Solid Edge part; units mm, degrees
sketch "Sketch1" plane through (0, 0, 0) normal (0, 0, 1) x (1, 0, 0)
  line L0 (-60, -45) -> (60, -45)
  line L1 (60, -45) -> (60, 45)
  line L2 (60, 45) -> (-60, 45)
  line L3 (-60, 45) -> (-60, -45)
extrude "Protrusion1" add sketch "Sketch1" along normal blind 15
sketch "Sketch2" plane through (0, 0, 0) normal (0, 0, -1) x (1, 0, 0)
  circle A0 centre (0, 0) radius 26
extrude "VaciadoExtruido_1" cut sketch "Sketch2" against normal blind 4
sketch "Sketch3" plane through (0, 0, 4) normal (0, 0, -1) x (1, 0, 0)
  line L0 (-12, -12) -> (12, -12)
  line L1 (12, -12) -> (12, 12)
  line L2 (12, 12) -> (-12, 12)
  line L3 (-12, 12) -> (-12, -12)
  dimension "D1" = 12
  dimension "D2" = 12
extrude "Cutout1" cut sketch "Sketch3" against normal through all
fillet "Redondeo_1" radius 2 4 edges at (-12, 12, 9.5) (-12, -12, 9.5) (12, -12, 9.5) (12, 12, 9.5)
chamfer "Chaflán_1" distance 5 angle 45 4 edges at (-60, 45, 7.5) (-60, -45, 7.5) (60, -45, 7.5) (60, 45, 7.5)
hole "Agujero_1" at (0, 38, 15) direction (0, 0, -1) diameter 8 end up to next start chamfer 0.5 start chamfer angle 45 end chamfer 0.5 end chamfer angle 45
hole "Hole1" at (0, -38, 15) direction (0, 0, -1) diameter 8 end up to next start chamfer 0.5 start chamfer angle 45 end chamfer 0.5 end chamfer angle 45
hole "Agujero_3" at (45.4585, 38, 15) direction (0, 0, -1) diameter 4.917 end through all start chamfer 0.5 start chamfer angle 45 end chamfer 0.5 end chamfer angle 45 thread major 6 thread length 2
hole "Hole2" at (43, -38, 15) direction (0, 0, -1) diameter 4.917 end through all start chamfer 0.5 start chamfer angle 45 end chamfer 0.5 end chamfer angle 45 thread major 6 thread length 2
hole "Hole3" at (-43, -38, 15) direction (0, 0, -1) diameter 4.917 end through all start chamfer 0.5 start chamfer angle 45 end chamfer 0.5 end chamfer angle 45 thread major 6 thread length 2
hole "Hole4" at (-43, 38, 15) direction (0, 0, -1) diameter 4.917 end through all start chamfer 0.5 start chamfer angle 45 end chamfer 0.5 end chamfer angle 45 thread major 6 thread length 2
Model file for the job. Use its own axes, mm. A direction names the side the tool comes from. Coordinates: 2 decimals unless noted, no trailing zeros. Write each loop counter-clockwise with the first axis right and the second up, starting at its lowest first coordinate (ties: lowest second). Pieces come first, ordered by that corner, then holes. Notation, with made-up numbers: (-4, 1.5) - (44, 1.5) arc R22 ccw to (44, 28.5) - close; hole circle Ø11 at (60.5, 63.5). An arc over 180 degrees is marked (long way). Use a Markdown table: item, result. Add a question column.
Item 1: Drop flat-ended pins along their axis: pin 1 (5.5 mm diameter, centred on x = -43, y = -38, fed in from +Z); pin 2 (3 mm diameter, centred on x = 43, y = -38, fed in from -Z). Give the stop position or say it passes through.
Item 2: Two-plate mould, pull along Y, no slides. Class faces 3 (the face through (-2.4, -34.8, 7.6)), 4 (the face through (58, -42, 8)), 5 (the face through (-57, 43, 7)): pulls with the +Y half, pulls with the -Y half, needs draft (parallel to the pull), parting line crosses it, or undercut.
Item 3: 3-axis set-ups, long thin cutter, end or side, ignore diameter. For faces 1 (the face through (1, 45, 7)), 2 (the face through (0, 12, 9)): which of +Z, -Z, +X, -X, +Y, -Y reach the whole face in a straight line?
Item 4: Band-saw the part on D-D, the plane x = -43. Write the cut outline in (y, z), and give its area (3 significant figures).
Item 5: Band-saw the part on B-B, the plane x = 0. Write the cut outline in (y, z), and give its area (3 significant figures).
Item 6: Band-saw the part on A-A, the plane y = 38. Write the cut outline in (x, z).
Item 7: Band-saw the part on C-C, the plane z = 13. Write the cut outline in (x, y).
Item 8: Drill centre lines: line 1 along X through (y, z) = (-38, 10.5); line 2 along X through (y, z) = (38, 10.5); line 3 along Y through (x, z) = (0, 4.75). Where is each one in solid material? Low to high.
A:
| question | item | result |
|---|---|---|
| 1 | pin 1 | stops at z = 14.79 |
| 1 | pin 2 | passes through |
| 2 | face 3 | undercut |
| 2 | face 4 | pulls with the -Y half |
| 2 | face 5 | pulls with the +Y half |
| 3 | face 1 | +Z, -Z, +X, -X, +Y |
| 3 | face 2 | +Z, -Z |
| 4 | outline | (-45, 0) - (-40.96, 0) - (-40.46, 0.5) - (-40.46, 14.5) - (-40.96, 15) - (-45, 15) - close; (-35.54, 0.5) - (-35.04, 0) - (35.04, 0) - (35.54, 0.5) - (35.54, 14.5) - (35.04, 15) - (-35.04, 15) - (-35.54, 14.5) - close; (40.46, 0.5) - (40.96, 0) - (45, 0) - (45, 15) - (40.96, 15) - (40.46, 14.5) - close |
| 4 | area | 1,200 mm² |
| 5 | outline | (-45, 0) - (-42.5, 0) - (-42, 0.5) - (-42, 14.5) - (-42.5, 15) - (-45, 15) - close; (-34, 0.5) - (-33.5, 0) - (-26, 0) - (-26, 4) - (-12, 4) - (-12, 15) - (-33.5, 15) - (-34, 14.5) - close; (12, 4) - (26, 4) - (26, 0) - (33.5, 0) - (34, 0.5) - (34, 14.5) - (33.5, 15) - (12, 15) - close; (42, 0.5) - (42.5, 0) - (45, 0) - (45, 15) - (42.5, 15) - (42, 14.5) - close |
| 5 | area | 637 mm² |
| 6 | outline | (-60, 0) - (-45.96, 0) - (-45.46, 0.5) - (-45.46, 14.5) - (-45.96, 15) - (-60, 15) - close; (-40.54, 0.5) - (-40.04, 0) - (-4.5, 0) - (-4, 0.5) - (-4, 14.5) - (-4.5, 15) - (-40.04, 15) - (-40.54, 14.5) - close; (4, 0.5) - (4.5, 0) - (42.5, 0) - (43, 0.5) - (43, 14.5) - (42.5, 15) - (4.5, 15) - (4, 14.5) - close; (47.92, 0.5) - (48.42, 0) - (60, 0) - (60, 15) - (48.42, 15) - (47.92, 14.5) - close |
| 7 | outline | (-60, -40) - (-55, -45) - (55, -45) - (60, -40) - (60, 40) - (55, 45) - (-55, 45) - (-60, 40) - close; hole circle Ø4.92 at (-43, -38); hole circle Ø4.92 at (-43, 38); hole (-12, -10) arc R2 ccw to (-10, -12) - (10, -12) arc R2 ccw to (12, -10) - (12, 10) arc R2 ccw to (10, 12) - (-10, 12) arc R2 ccw to (-12, 10) - close; hole circle Ø8 at (0, -38); hole circle Ø8 at (0, 38); hole circle Ø4.92 at (43, -38); hole circle Ø4.92 at (45.46, 38) |
| 8 | line 1 | x = -60 to -45.46, -40.54 to -4, 4 to 40.54, 45.46 to 60 |
| 8 | line 2 | x = -60 to -45.46, -40.54 to -4, 4 to 43, 47.92 to 60 |
| 8 | line 3 | y = -45 to -42, -34 to -12, 12 to 34, 42 to 45 |
